Part print with two shaded views. Sizes in mm from the minimum x, y, z corner. A direction names the side the tool comes from. Round coordinates to 2 decimals unless told otherwise and drop trailing zeros. Order: outer loops, then holes, each group sorted by start corner. A loop starts at its lowest first (then second) coordinate and runs counter-clockwise, first axis right, second up. Notation, with made-up numbers: (67, -12) -> (104, -12) arc R11 ccw to (104, 1) -> close; hole circle Ø2 at (83, 79). An arc over 180 degrees is marked (long way). Put each result on its own line as item: value. Start each with the question number.
Q1. Cut at B-B, the plane z = 20.5. List the corners of the cut face in (x, y).
Q2. 3-axis set-ups, long thin cutter, end or side, ignore diameter. For the marked faces 1 and 2: which of +Z, -Z, +X, -X, +Y, -Y reach the whole face in a straight line?
Q3. Pull direction X, two halves, no side cores. Call the marked faces 3, 4 and 5: released by +X, released by -X, zero draft, split by the parting line, or undercut.
Q4. Cut at D-D, the plane x = 5.5. List the corners of the cut face in (y, z), and give its area (3 significant figures).
Q5. Flat gauge pins, fed straight in: P1, Ø1, axis at x = 6.5, y = 16.5, coming from the +Z side; P2, Ø16, axis at x = 15, z = 19, coming from the -Y side. Where does each tip first touch, or does it go through?
Q6. Probe L1, parallel to Y at x = 15, z = 0.6; L2, parallel to Z at x = 15, y = 28; L3, parallel to Y at x = 28.5, z = 6. List the from-to ranges inside material, lowest first.
Q7. Cut at A-A, the plane y = 15. List the corners of the cut face in (x, z), and give its area (4 significant figures).
Q8. Cut at C-C, the plane y = 8.5. List the corners of the cut face in (x, z), and give its area (3 significant figures).
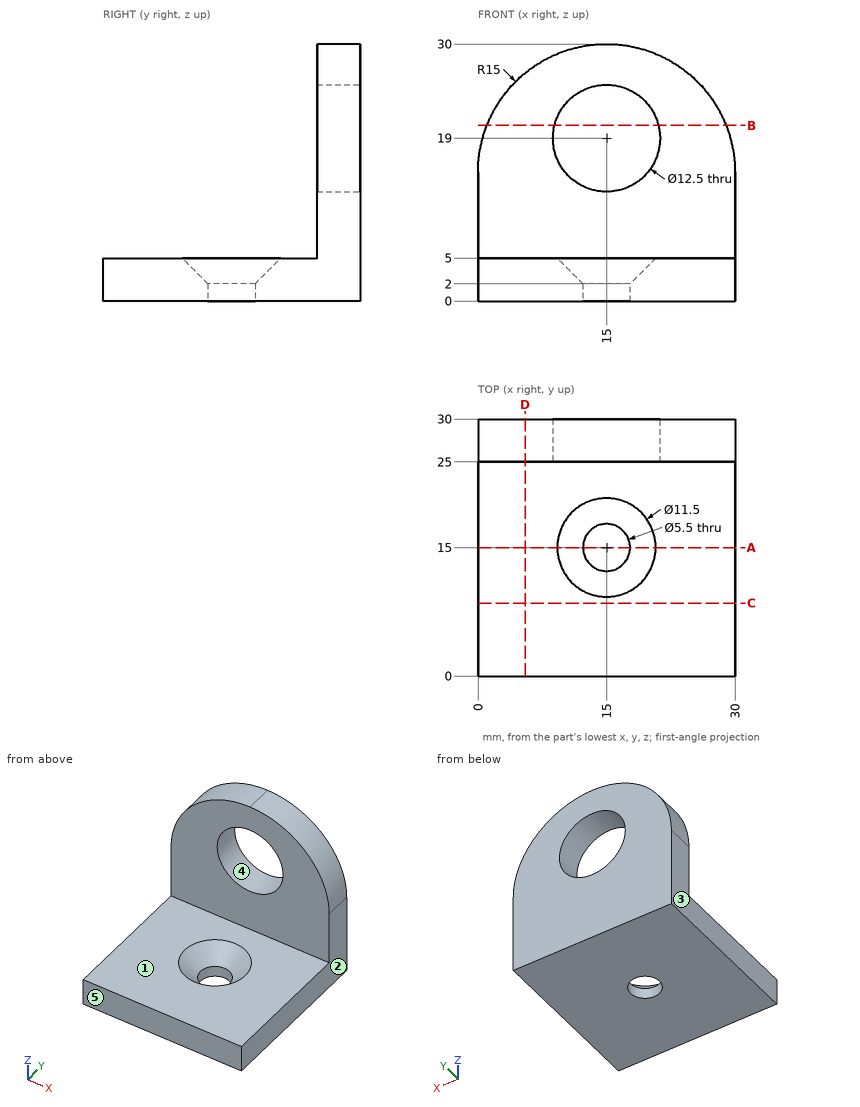
Ans:
1. outline: (1.04, 25) -> (8.93, 25) -> (8.93, 30) -> (1.04, 30) -> close; (21.07, 25) -> (28.96, 25) -> (28.96, 30) -> (21.07, 30) -> close
2. face 1: +Z, +X, -X, -Y
2. face 2: +Z, -Z, +X, +Y, -Y
3. face 3: released by -X
3. face 4: undercut
3. face 5: zero draft
4. outline: (0, 0) -> (30, 0) -> (30, 26.61) -> (25, 26.61) -> (25, 5) -> (0, 5) -> close
4. area: 258 mm^2
5. P1: stops at z = 5
5. P2: stops at y = 25
6. L1: y = 0 to 12.25, 17.75 to 30
6. L2: z = 0 to 12.75, 25.25 to 30
6. L3: y = 25 to 30
7. outline: (0, 0) -> (12.25, 0) -> (12.25, 2) -> (9.25, 5) -> (0, 5) -> close; (17.75, 0) -> (30, 0) -> (30, 5) -> (20.75, 5) -> (17.75, 2) -> close
7. area: 113.5 mm^2
8. outline: (0, 0) -> (30, 0) -> (30, 5) -> (0, 5) -> close
8. area: 150 mm^2
